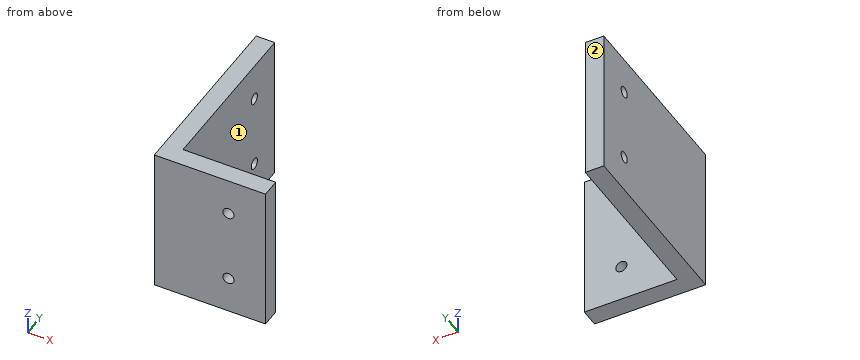
Autodesk Inventor part; units mm, degrees
ref_plane "YZ Plane" through (0, 0, 0) normal (1, 0, 0) x (0, 1, 0)
ref_plane "XZ Plane" through (0, 0, 0) normal (0, 1, 0) x (-1, 0, 0)
ref_plane "XY Plane" through (0, 0, 0) normal (0, 0, 1) x (1, 0, 0)
sketch "Sketch1" plane through (0, 0, 0) normal (0, 0, 1) x (1, 0, 0)
  line L0 (0, 0) -> (0, 50)
  line L1 (0, 50) -> (5, 50)
  line L2 (5, 50) -> (5, 5)
  line L3 (5, 5) -> (30, 5)
  line L4 (30, 5) -> (30, 0)
  line L5 (30, 0) -> (0, 0)
  dimension "d0" = 50
  dimension "d1" = 5
  dimension "d2" = 45
  dimension "d3" = 25
  dimension "d4" = 5
extrude "Extrusion1" add sketch "Sketch1" along normal blind 40
sketch "Sketch2" plane through (0, 0, 0) normal (-1, 0, 0) x (0, 0, 1)
  circle A0 centre (10, 40) radius 1.5
  circle A1 centre (30, 40) radius 1.5
  point P0 (0, 0)
  dimension "d7" = 3
  dimension "d8" = 3
sketch "Sketch3" plane through (0, 0, 0) normal (-1, 0, 0) x (0, 0, 1)
  point P0 (0, 0)
extrude "Extrusion2" cut sketch "Sketch2" against normal through all
sketch "Sketch4" plane through (5, 5, 0) normal (0, 1, 0) x (1, 0, 0)
  point P0 (-5, 0)
sketch "Sketch5" plane through (0, 0, 0) normal (0, -1, 0) x (1, 0, 0)
  circle A0 centre (20, 30) radius 1.5
  circle A1 centre (20, 10) radius 1.5
  point P0 (0, 0)
  dimension "d11" = 3
  dimension "d12" = 3
extrude "Extrusion3" cut sketch "Sketch5" against normal through all
properties part number "moter support"
Could you check a few things on this model? Use its own coordinates, in mm. Face numbers are marked on the shaded views. A direction names the side the tool comes from. Give positions to 0.01 mm unless a question says otherwise; leave off trailing zeros. Order: outer loops, then holes, each group sorted by start corner. A loop starts at its lowest first (then second) coordinate and runs counter-clockwise, first axis right, second up.
Q1. I'm going to push flat-ended pins straight in: P1, Ø12.5, axis at x = 15, z = 18.5, coming from the +Y side; P2, Ø1.8, axis at x = 20, z = 30, coming from the -Y side; P3, Ø1.5, axis at y = 8, z = 29, coming from the +X side. Where does each tip first touch, or does it pass through?
Q2. For the marked faces 1 and 2, which set-ups out of +Z, -Z, +X, -X, +Y, -Y let a thin tool reach every point of the face, with its end or its side?
Q3. If I drill on line 1 along Z through (x, y) = (20, 1.15); line 2 along Y through (x, z) = (3.55, 10); line 3 along X through (y, z) = (42.5, 27), over which ranges is the centre line in solid material (lowest first)?
Q4. Suppose I cut it at D-D, the plane z = 26. Write out the boundary of the cut face in (x, y), and give its area (3 significant figures).
Q5. Suppose I cut it at A-A, the plane z = 10. Write out the boundary of the cut face in (x, y), and give its area (3 significant figures).
Q6. Suppose I cut it at B-B, the plane y = 40. Write out the boundary of the cut face in (x, z).
Solution:
1. P1: stops at y = 5
1. P2: passes through
1. P3: stops at x = 5
2. face 1: +Z, -Z, +X, +Y
2. face 2: +Z, -Z, +X, -X, +Y
3. line 1: z = 0 to 8.5, 11.5 to 28.5, 31.5 to 40
3. line 2: y = 0 to 38.5, 41.5 to 50
3. line 3: x = 0 to 5
4. outline: (0, 0) - (30, 0) - (30, 5) - (5, 5) - (5, 50) - (0, 50) - close
4. area: 375 mm2
5. outline: (0, 0) - (18.5, 0) - (18.5, 5) - (5, 5) - (5, 38.5) - (0, 38.5) - close; (0, 41.5) - (5, 41.5) - (5, 50) - (0, 50) - close; (21.5, 0) - (30, 0) - (30, 5) - (21.5, 5) - close
5. area: 345 mm2
6. outline: (0, 0) - (5, 0) - (5, 8.5) - (0, 8.5) - close; (0, 11.5) - (5, 11.5) - (5, 28.5) - (0, 28.5) - close; (0, 31.5) - (5, 31.5) - (5, 40) - (0, 40) - close
